Can you work these out from the model? Positions are in its coordinate system, mm. A direction names the side the tool comes from. Round coordinates to 2 decimals unless told otherwise and drop trailing zeros. Order: outer loops, then holes, each group sorted by start corner. A loop starts at its lowest first (then second) coordinate and runs counter-clockwise, first axis right, second up. Notation, with made-up numbers: M 0,59.25 L 20,59.25 A18 cw 20,82.25 Z; hole C -11,34.25 d8. An arc over 180 degrees is marked long. One line per question, with ' | ' between items.
```python
from build123d import *

# Parameters (mm, degrees)
F1_DEPTH = 9.525
F3_W     = 87.0458
F3_H     = 63.5
F3_W_2   = 38.1
F3_H_2   = 12.7
F4_DEPTH = 9.525
F6_DEPTH = 4.7625


with BuildPart() as f1:
    # F0 (on Right) → F1 (new body)
    with BuildSketch(Plane.YZ):
        Polygon((-127, 63.5), (-25.4, 63.5), (-25.4, 127), (-44.45, 127), (-76.2, 95.25), (-107.95, 127), (-127, 127), align=None)
    extrude(amount=F1_DEPTH)


with BuildPart() as f1_1:
    # F2: moved
    add(f1.part.moved(Location((25.4, 88.9, 0))))

    # F3 (on face) → F4 (join)
    with BuildSketch(Plane.YZ.offset(34.925)):
        with Locations((107.0229, 136.525)):
            Rectangle(F3_W, F3_H)
        with Locations((-19.05, 57.15)):
            Rectangle(F3_W_2, F3_H_2)
    extrude(amount=-F4_DEPTH)

    # F5 (on face) → F6 (join)
    with BuildSketch(Plane.XY.offset(168.275)):
        Polygon((6.5405, 150.5458), (6.5405, 108.204), (53.7845, 108.204), (53.7845, 129.3749), (53.7845, 150.5458), align=None)
        with BuildLine():
            Line((53.7845, 108.204), (6.5405, 108.204))
            Line((6.5405, 108.204), (6.534646, 101.854003))
            Line((6.534646, 101.854003), (15.267185, 101.854003))
            ThreePointArc((15.267185, 101.854003), (30.1625, 106.68), (45.057815, 101.854003))
            Line((45.057815, 101.854003), (55.5625, 101.854003))
            Line((55.5625, 101.854003), (55.5625, 38.354))
            Line((55.5625, 38.354), (74.6125, 38.354))
            Line((74.6125, 38.354), (74.6125, 108.5469))
            Line((74.6125, 108.5469), (53.7845, 129.3749))
            Line((53.7845, 129.3749), (53.7845, 108.204))
        make_face()
    extrude(amount=F6_DEPTH)


solid = f1_1.part
```
(1) If we section it at A-A on z = 114: Please give me the cut outline in (x, y) (3 decimals).
Final values:
outline: M 25.4,-38.1 L 34.925,-38.1 L 34.925,-6.05 L 25.4,-6.05 Z; M 25.4,31.45 L 34.925,31.45 L 34.925,150.546 L 25.4,150.546 Z
(2) Please list where these lines run through material, in increasing order: probe 1 along Z at (x, y) = (70, 94) (1 decimal); probe 2 along X at (y, z) = (70.5, 164.5) (3 decimals); probe 3 along Y at (x, z) = (32.5, 86). Write a range as [from, to].
Final values:
probe 1: [168.3, 173] | probe 2: [25.4, 34.925] | probe 3: [-38.1, 63.5]
(3) If we section it at B-B on y = 86: Please give me the cut outline in (x, z) (1 decimal).
Final values:
outline: M 25.4,104.8 L 34.9,104.8 L 34.9,168.3 L 25.4,168.3 Z; M 55.6,168.3 L 74.6,168.3 L 74.6,173 L 55.6,173 Z
(4) Will these pins go through, and if not, where does the flat tip stop? pin 1 Ø5 at (y, z) = (48, 124.5) entering from -X; pin 2 Ø5 at (x, z) = (66, 170.5) entering from -Y; pin 3 Ø5 at (x, y) = (28.5, 95.5) entering from +Z (3 decimals).
Final values:
pin 1: x = 25.4 | pin 2: y = 38.35 | pin 3: z = 168.275
(5) On a 3-axis mill with a long thin cutter (end or side, diameter ignored), from which of +Z, -Z, +X, -X, +Y, -Y can I reach the whole of each face in a straight line? I mean faces 1 (the flat face through (16, 127, 168.275)), 2 (the flat face through (30, 54, 127)), 3 (the flat face through (30, 63.5, 84)), 4 (the flat face through (34.925, 55, 110)). Say none if no direction works.
Final values:
face 1: -Z, -X, +Y, -Y | face 2: +Z, +X, -X, -Y | face 3: -Z, +X, -X, +Y | face 4: -Z, +X, +Y, -Y
(6) Thinking about a two-plate mould opening in Y: for faces 5 (the flat face through (64.34, 118.82, 170.62)), 6 (the flat face through (30.1, 28.8, 111.35)), 7 (the flat face through (59, 95, 168.275)), which applies, released by +Y, released by -Y, zero draft, split by the parting line, or undercut?
Final values:
face 5: released by +Y | face 6: undercut | face 7: zero draft
(7) If we section it at C-C on y = 137: Please give me the cut outline in (x, z) (1 decimal).
Final values:
outline: M 6.5,168.3 L 25.4,168.3 L 25.4,104.8 L 34.9,104.8 L 34.9,168.3 L 53.8,168.3 L 53.8,173 L 6.5,173 Z
